```python
from build123d import *

# Parameters (mm, degrees)
EXTRUDE_1_DEPTH     = 0.4
SKETCH_3_W          = 2.5
SKETCH_3_H          = 2.5
EXTRUDE_2_DEPTH     = 1.5
CUT_EXTRUDE_1_REACH = 27.763
SKETCH_5_R          = 1
EXTRUDE_START       = -0.4
SKETCH_6_R          = 3.65
EXTRUDE_3_DEPTH     = 9


with BuildPart() as part:
    # 草图1 → 凸台-拉伸1 (new body)
    with BuildSketch(Plane(origin=(0, 0, 0), x_dir=(1, 0, 0), z_dir=(0, 1, 0))):
        with BuildLine():
            Line((-2.5, 12.528839135), (-2.5, 23.978839135))
            Line((-2.5, 23.978839135), (2.5, 23.978839135))
            Line((2.5, 23.978839135), (2.5, 12.528839135))
            ThreePointArc((2.5, 12.528839135), (7.407428704, 9.194327232), (9.3, 3.571160865))
            Line((9.3, 3.571160865), (9.3, -3.571160865))
            Line((9.3, -3.571160865), (-9.3, -3.571160865))
            Line((-9.3, -3.571160865), (-9.3, 3.571160865))
            ThreePointArc((-9.3, 3.571160865), (-7.407428704, 9.194327232), (-2.5, 12.528839135))
        make_face()
    extrude(amount=EXTRUDE_1_DEPTH)

    # 草图3 → 凸台-拉伸2 (add)
    with BuildSketch(Plane.XZ):
        with Locations((7.55, -2.278839135)):
            Rectangle(SKETCH_3_W, SKETCH_3_H)
        with Locations((-7.55, -2.278839135)):
            Rectangle(SKETCH_3_W, SKETCH_3_H)
    extrude(amount=EXTRUDE_2_DEPTH)

    # 草图5 → 切除-拉伸1 (cut, up to next)
    with BuildSketch(Plane.XZ, mode=Mode.PRIVATE) as cut_extrude_1_sk1:
        with Locations(Location((0, -20.978839135, 0), (0, 0, 270))):
            Circle(SKETCH_5_R)
    cut_extrude_1_tool1 = extrude(cut_extrude_1_sk1.sketch, amount=-CUT_EXTRUDE_1_REACH, mode=Mode.PRIVATE) & part.part
    add(cut_extrude_1_tool1.solids().sort_by_distance((0, 0, -20.978839))[0], mode=Mode.SUBTRACT)

    # 草图6 → 凸台-拉伸3 (add)
    with BuildSketch(Plane.XZ.offset(EXTRUDE_START)):
        with Locations(Location((0, -3.571160865, 0), (0, 0, 270))):
            Circle(SKETCH_6_R)
    extrude(amount=EXTRUDE_3_DEPTH)


solid = part.part
```
Source: CAD feature listing. Evaluate the final solid. Frame: model axes, mm. A direction names the side the tool comes from. Give positions to 0.01 mm unless a question says otherwise; leave off trailing zeros. Order: outer loops, then holes, each group sorted by start corner. A loop starts at its lowest first (then second) coordinate and runs counter-clockwise, first axis right, second up. Notation, with made-up numbers: (39, -39.75) -> (77, -39.75) arc R28 cw to (77, -0.75) -> close; hole circle Ø1 at (1, 11). An arc over 180 degrees is marked (long way). Use a Markdown table: item, result.
Q1. Section B-B (y = -0.5). Return the cut outline in (x, z), and give its area (3 significant figures).
A:
| item | result |
|---|---|
| outline | (-8.8, -3.53) -> (-6.3, -3.53) -> (-6.3, -1.03) -> (-8.8, -1.03) -> close; circle Ø7.3 at (0, -3.57); (6.3, -3.53) -> (8.8, -3.53) -> (8.8, -1.03) -> (6.3, -1.03) -> close |
| area | 54.4 mm^2 |
Q2. Material intervals for line 1 (Y direction, x = -6.25, z = 0.25); line 2 (Y direction, x = -8.25, z = -2.25); line 3 (Z direction, x = 8, y = -0.25), sorted ascending. Write a range as [from, to].
A:
| item | result |
|---|---|
| line 1 | [0, 0.4] |
| line 2 | [-1.5, 0.4] |
| line 3 | [-3.53, -1.03] |
Q3. Section D-D (y = -7.75). Return the cut outline in (x, z).
A:
| item | result |
|---|---|
| outline | circle Ø7.3 at (0, -3.57) |
Q4. First-contact query: P1, Ø0.8, axis at y = -1, z = -2.5, coming from the -X side; P2, Ø2, axis at x = -7, z = -2, coming from the -Y side; P3, Ø4, axis at y = -7.5, z = -5, coming from the +X side. Flat tips, straight axial feed; report the tip coordinate or a pass-through.
A:
| item | result |
|---|---|
| P1 | x = -8.8 |
| P2 | y = -1.5 |
| P3 | x = 3.65 |
Q5. Section C-C (z = -17). Return the cut outline in (x, y), and give its area (3 significant figures).
A:
| item | result |
|---|---|
| outline | (-2.5, 0) -> (2.5, 0) -> (2.5, 0.4) -> (-2.5, 0.4) -> close |
| area | 2.00 mm^2 |
Q6. Pull-direction query (X, two-part tool) for faces 1 (the face through (-8, -1.5, -2)), 2 (the face through (-6.3, -1, -2)), 3 (the face through (0.04, 0.2, -19.98)), 4 (the face through (-7.458, 0.197, -9.127)); classes: +X half, -X half, draft (parallel to the pull), parting line (faces both ways), or undercut.
A:
| item | result |
|---|---|
| face 1 | draft |
| face 2 | undercut |
| face 3 | undercut |
| face 4 | -X half |
Q7. Section A-A (x = 0). Return the cut outline in (y, z).
A:
| item | result |
|---|---|
| outline | (-8.6, -7.22) -> (0, -7.22) -> (0, -19.98) -> (0.4, -19.98) -> (0.4, 3.57) -> (0, 3.57) -> (0, 0.08) -> (-8.6, 0.08) -> close; (0, -23.98) -> (0.4, -23.98) -> (0.4, -21.98) -> (0, -21.98) -> close |
Q8. Access query for faces 5 (the face through (-8, -1, -3.529)), 6 (the face through (8, -1.5, -2)), 7 (the face through (8, -1, -1.029)), 8 (the face through (-8.8, -1, -2)). Directions: +Z, -Z, +X, -X, +Y, -Y. A direction counts if a zero-diameter tool reaches every point of the face in a straight line with its end or side. Return the directions, or none.
A:
| item | result |
|---|---|
| face 5 | -Z, -X, -Y |
| face 6 | +Z, -Z, +X, -Y |
| face 7 | +Z, +X, -Y |
| face 8 | +Z, -Z, -X, -Y |
